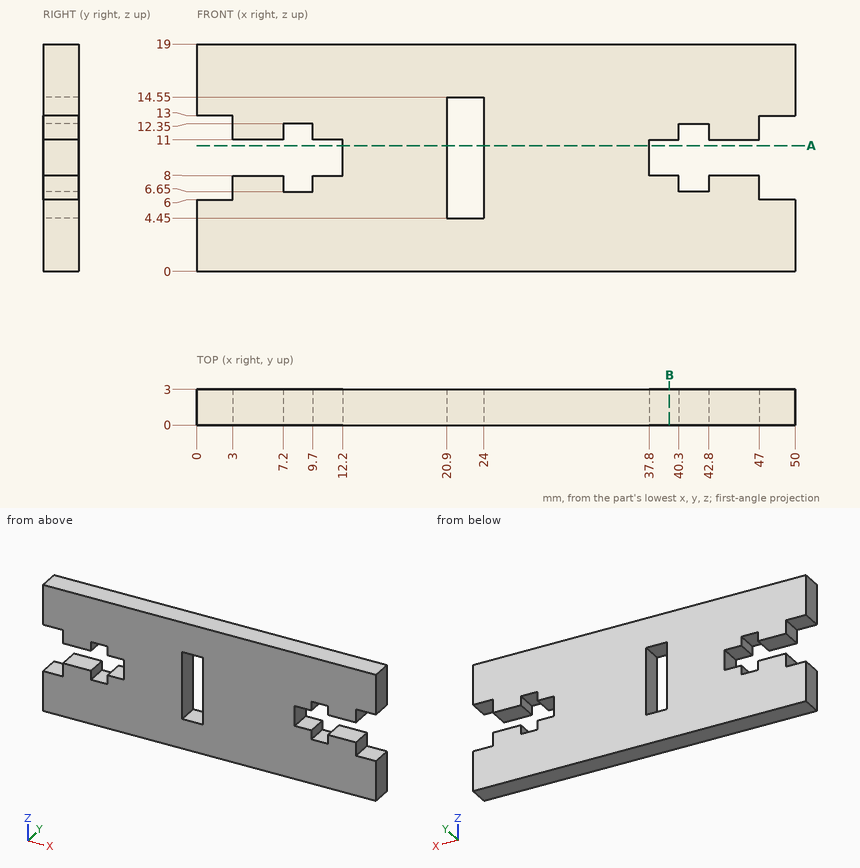
Geometry check sheet. Reference: drawing and pictorial views, mm from the part's lowest x, y, z. Round coordinates to 2 decimals unless told otherwise and drop trailing zeros. Write each loop counter-clockwise with the first axis right and the second up, starting at its lowest first coordinate (ties: lowest second). Pieces come first, ordered by that corner, then holes.
Item 1: Material ranges on line 1 along X through (y, z) = (2.2, 6.75); line 2 along X through (y, z) = (2.4, 9.25); line 3 along Z through (x, y) = (4, 0.9), recorded low to high.
Determined:
line 1: x = 3 to 7.2, 9.7 to 20.9, 24 to 40.3, 42.8 to 47
line 2: x = 12.2 to 20.9, 24 to 37.8
line 3: z = 0 to 8, 11 to 19
Item 2: Go/stop test with flat-tipped pins: pin 1 Ø1 at (x, z) = (13.5, 7.5) entering from -Y; pin 2 Ø1 at (y, z) = (1, 7) entering from -X; pin 3 Ø0.9 at (y, z) = (1.5, 8.5) entering from +X. Record where each tip stops, or that it passes through.
Determined:
pin 1: stops at y = 0
pin 2: stops at x = 3
pin 3: stops at x = 37.8
Item 3: Section check A-A (z = 10.5). Record the boundary of the cut face in (x, y).
Determined:
outline: (12.2, 0) - (20.9, 0) - (20.9, 3) - (12.2, 3) - close; (24, 0) - (37.8, 0) - (37.8, 3) - (24, 3) - close
Item 4: Section check B-B (x = 39.5). Record the boundary of the cut face in (y, z).
Determined:
outline: (0, 0) - (3, 0) - (3, 8) - (0, 8) - close; (0, 11) - (3, 11) - (3, 19) - (0, 19) - close
